Can you work these out from the drawing? Everything is in mm from the part's minimum corner. A direction names the side the tool comes from. Give positions to 0.01 mm unless a question says otherwise; leave off trailing zeros. Order: outer loops, then holes, each group sorted by start corner. A loop starts at its lowest first (then second) coordinate and runs counter-clockwise, first axis right, second up. Notation, with made-up numbers: M 39,-10 L 68,-10 A30 cw 68,19 Z; hole C 8.25,10.5 d4. An arc over 180 degrees is marked long. Answer as a JSON object with one key per item and string values.
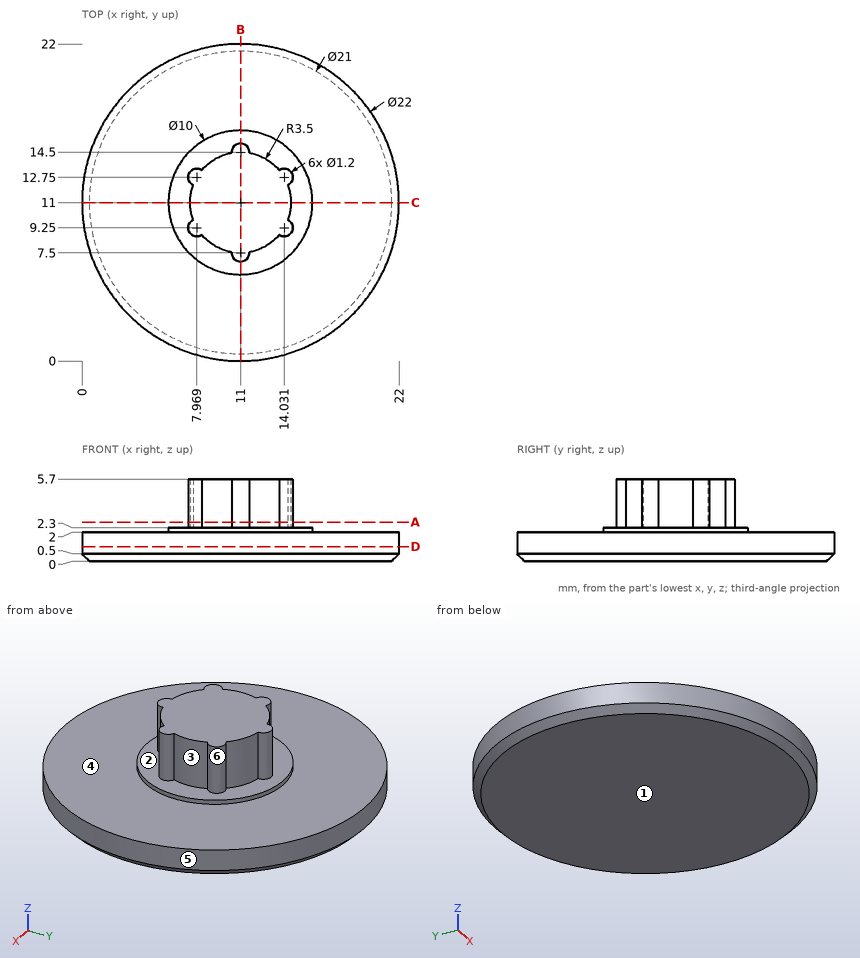
1) Thinking about a two-plate mould opening in Y: for the marked faces 4, 5 and 6, which applies, pulls with the +Y half, pulls with the -Y half, needs draft (parallel to the pull), parting line crosses it, or undercut?
Results found:
{"face 4": "needs draft", "face 5": "parting line crosses it", "face 6": "undercut"}
2) I want a section at D-D on z = 1. Write out the boundary of the cut face in (x, y), and give its area (3 significant figures).
Results found:
{"outline": "C 11,11 d22", "area": "380 mm²"}
3) I'm going to push flat-ended pins straight in: pin 1 Ø3 at (x, y) = (10.5, 15) entering from +Z; pin 2 Ø1 at (x, z) = (16, 1.5) entering from -Y; pin 3 Ø3 at (x, y) = (4.5, 14.5) entering from +Z. Where does each tip first touch, or does it pass through?
Results found:
{"pin 1": "stops at z = 5.7", "pin 2": "stops at y = 0.96", "pin 3": "stops at z = 2"}
4) I need wall thicknesses on L1, parallel to Z at x = 15.25, y = 7.75; L2, parallel to Y at x = 8.75, z = 5.1; L3, parallel to X at y = 9.5, z = 0.4. Which ranges of each line are inside material? Lowest first, please.
Results found:
{"L1": "z = 0 to 2", "L2": "y = 8.32 to 13.68", "L3": "x = 0.2 to 21.8"}
5) I want a section at A-A on z = 2.7. Write out the boundary of the cut face in (x, y), and give its area (3 significant figures).
Results found:
{"outline": "M 7.71,9.79 A0.6 ccw long 8.31,8.76 A3.5 ccw 10.4,7.55 A0.6 ccw long 11.6,7.55 A3.5 ccw 13.69,8.76 A0.6 ccw long 14.29,9.79 A3.5 ccw 14.29,12.21 A0.6 ccw long 13.69,13.24 A3.5 ccw 11.6,14.45 A0.6 ccw long 10.4,14.45 A3.5 ccw 8.31,13.24 A0.6 ccw long 7.71,12.21 A3.5 ccw Z", "area": "42.0 mm²"}
6) I want a section at C-C on y = 11. Write out the boundary of the cut face in (x, z).
Results found:
{"outline": "M 0,0.5 L 0.5,0 L 21.5,0 L 22,0.5 L 22,2 L 16,2 L 16,2.3 L 14.5,2.3 L 14.5,5.7 L 7.5,5.7 L 7.5,2.3 L 6,2.3 L 6,2 L 0,2 Z"}
7) I want a section at B-B on x = 11. Write out the boundary of the cut face in (y, z), and give its area (3 significant figures).
Results found:
{"outline": "M 0,0.5 L 0.5,0 L 21.5,0 L 22,0.5 L 22,2 L 16,2 L 16,2.3 L 15.1,2.3 L 15.1,5.7 L 6.9,5.7 L 6.9,2.3 L 6,2.3 L 6,2 L 0,2 Z", "area": "74.6 mm²"}
8) For the marked faces 1, 2 and 3, which set-ups out of +Z, -Z, +X, -X, +Y, -Y let a thin tool reach every point of the face, with its end or its side?
Results found:
{"face 1": "-Z, +X, -X, +Y, -Y", "face 2": "+Z", "face 3": "+Z, +X"}
